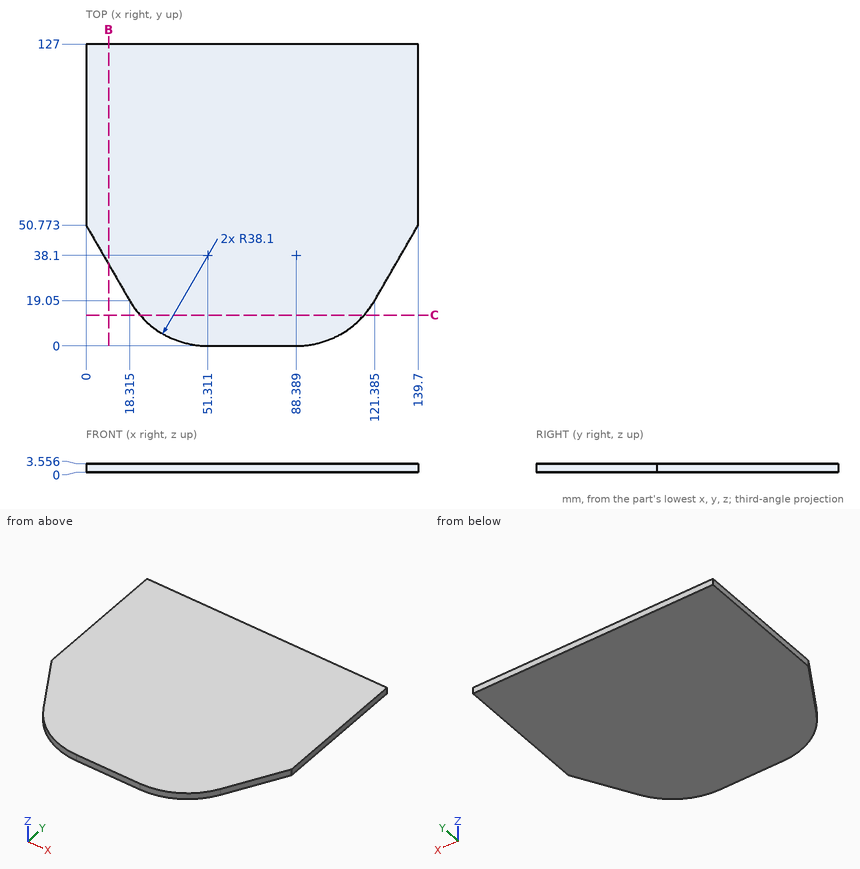
Source: three-view drawing plus pictorial views. Frame: mm from the lowest corner of the part. Round coordinates to 2 decimals unless told otherwise and drop trailing zeros. Order: outer loops, then holes, each group sorted by start corner. A loop starts at its lowest first (then second) coordinate and runs counter-clockwise, first axis right, second up. Notation, with made-up numbers: (-31.75, -1) -> (5.25, -1) arc R20 ccw to (5.25, 16) -> close; hole circle Ø3 at (58, -7.5). An arc over 180 degrees is marked (long way). Use one line per item in the form item = value.
(1) Section B-B on x = 9.5. Return loops of the section in (y, z).
Results list:
outline = (34.32, 0) -> (127, 0) -> (127, 3.56) -> (34.32, 3.56) -> close
(2) Ray query, probe 1 along X at (y, z) = (38.5, 0.95) (1 decimal); probe 2 along Y at (x, z) = (104, 0.85) (1 decimal); probe 3 along Y at (x, z) = (44, 0.7). Return the intervals inside material, ascending. Write a range as [from, to].
Results list:
probe_1 = [7.1, 132.6]
probe_2 = [3.3, 127]
probe_3 = [0.71, 127]
(3) Section C-C on y = 13. Return loops of the section in (x, z).
Results list:
outline = (22.65, 0) -> (117.05, 0) -> (117.05, 3.56) -> (22.65, 3.56) -> close
(4) First-contact query: pin 1 Ø10 at (x, y) = (52.5, 95.5) entering from -Z; pin 2 Ø1 at (y, z) = (19, 0.5) entering from -X (1 decimal). Flat tips, straight axial feed; report the tip coordinate or a pass-through.
Results list:
pin_1 = 0
pin_2 = 18.1
